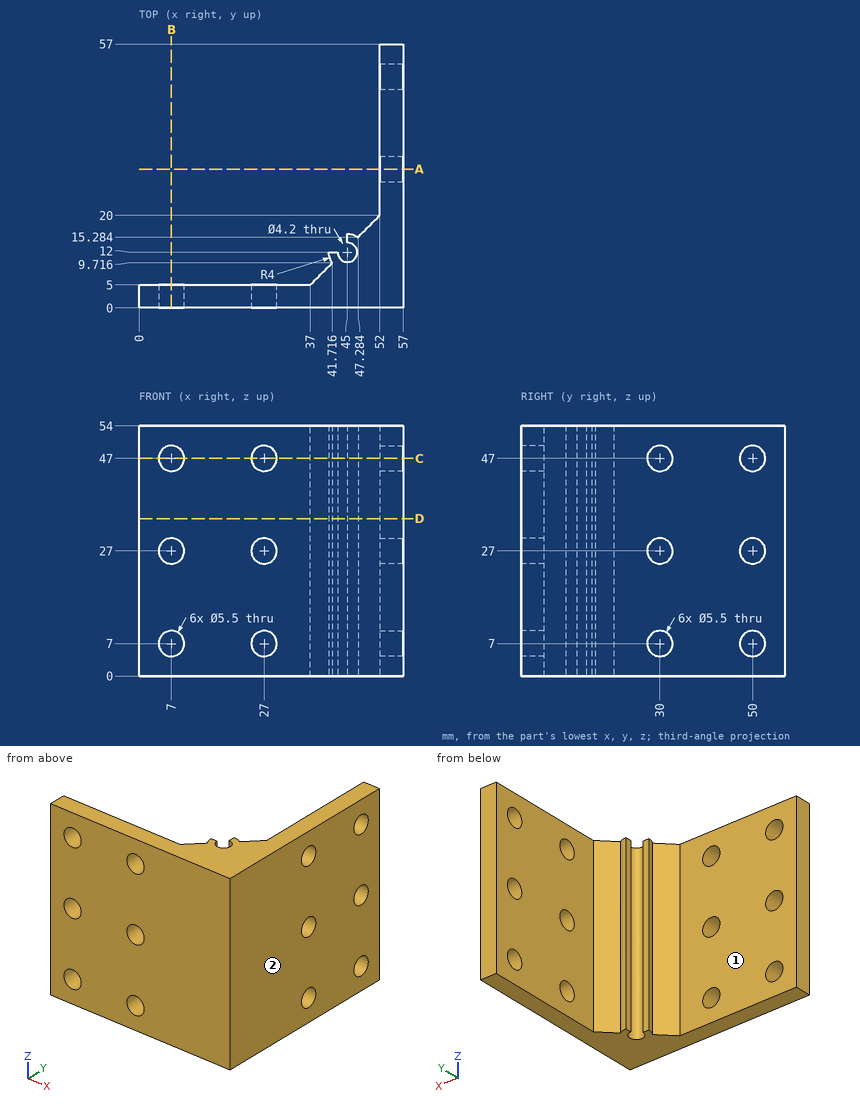
Study the drawing (mm; zero at the part's minimum x, y, z) and answer. A direction names the side the tool comes from. Coordinates: 2 decimals unless noted, no trailing zeros. Write each loop counter-clockwise with the first axis right and the second up, starting at its lowest first coordinate (ties: lowest second). Pieces come first, ordered by that corner, then holes. Notation, with made-up numbers: (77, 54.5) - (115, 54.5) arc R33 cw to (115, 92.5) - close; hole circle Ø10 at (50.25, -18.75). An arc over 180 degrees is marked (long way). Return JSON: item names as keys, results as strings. Group by question number.
1. A cutting plane is placed at C-C, the plane z = 47. Give the number of separate pieces and of enclosed holes in the cut face, plus the area to 3 significant figures.
2. Given pin 1 (3.5 mm diameter, centred on x = 7, z = 27, fed in from +Y); pin 2 (6.5 mm diameter, centred on y = 30, z = 7, fed in from -X); pin 3 (2 mm diameter, centred on x = 42, z = 26.5, fed in from +Y); pin 4 (1 mm diameter, centred on y = 15.5, z = 26, fed in from -X), each flat-ended and moving along its own axis, determine where each tip first touches the part or whether it passes through.
3. Straight lines are drawn through the part: L1, parallel to Y at x = 55, z = 47; L2, parallel to Z at x = 27, y = 4; L3, parallel to Z at x = 53.5, y = 32. For each, find the intervals that lie inside material, in ascending order.
4. Which of the six approach directions +Z, -Z, +X, -X, +Y, -Y give full straight-line access (tool end or side, diameter ignored) to the marked faces 1 and 2?
5. A cutting plane is placed at D-D, the plane z = 34. Determine the outline of the cut face in (x, y), plus the area to 3 significant figures.
6. A cutting plane is placed at A-A, the plane y = 30. Determine the outline of the cut face in (x, z), plus the area to 4 significant figures.
7. A cutting plane is placed at B-B, the plane x = 7. Determine the outline of the cut face in (y, z), plus the area to 4 significant figures.
Ans:
{
 "1": {"separate pieces": "5", "enclosed holes": "0", "area": "544 mm²"},
 "2": {"pin 1": "through", "pin 2": "x = 52", "pin 3": "y = 12", "pin 4": "x = 45"},
 "3": {"L1": "0 to 27.25, 32.75 to 47.25, 52.75 to 57", "L2": "0 to 4.25, 9.75 to 24.25, 29.75 to 44.25, 49.75 to 54", "L3": "0 to 5.11, 8.89 to 25.11, 28.89 to 45.11, 48.89 to 54"},
 "4": {"face 1": "+Z, -Z, -X, +Y", "face 2": "+Z, -Z, +X, +Y, -Y"},
 "5": {"outline": "(0, 0) - (57, 0) - (57, 57) - (52, 57) - (52, 20) - (47.28, 15.28) arc R4 ccw to (45, 16) - (45, 14.1) arc R2.1 cw (long way) to (42.9, 12) - (41, 12) arc R4 ccw to (41.72, 9.72) - (37, 5) - (0, 5) - close", "area": "654 mm²"},
 "6": {"outline": "(52, 0) - (57, 0) - (57, 4.25) - (52, 4.25) - close; (52, 9.75) - (57, 9.75) - (57, 24.25) - (52, 24.25) - close; (52, 29.75) - (57, 29.75) - (57, 44.25) - (52, 44.25) - close; (52, 49.75) - (57, 49.75) - (57, 54) - (52, 54) - close", "area": "187.5 mm²"},
 "7": {"outline": "(0, 0) - (5, 0) - (5, 4.25) - (0, 4.25) - close; (0, 9.75) - (5, 9.75) - (5, 24.25) - (0, 24.25) - close; (0, 29.75) - (5, 29.75) - (5, 44.25) - (0, 44.25) - close; (0, 49.75) - (5, 49.75) - (5, 54) - (0, 54) - close", "area": "187.5 mm²"}
}
